The listing builds one solid part. Answer for the finished solid, in the listing's coordinates (mm). A direction names the side the tool comes from. Give positions to 0.01 mm unless a question says otherwise; leave off trailing zeros. Loops run counter-clockwise (first coordinate to the right, second up) from the corner with the lowest first, then second, coordinate; pieces in that order, holes last. Notation, with made-up numbers: (15, -13) - (49, -13) arc R19 ccw to (49, -2) - close; hole circle Ø7 at (-6, -32). An arc over 180 degrees is marked (long way). Write each question's results on one line, items separated by ' | '.
from build123d import *

# Parameters (mm, degrees)
SKETCH3_W           = 60
SKETCH3_H           = 80
SKETCH3_R           = 1
SKETCH3_R_2         = 1.5
SKETCH3_W_2         = 22
SKETCH3_H_2         = 45
BOSS_EXTRUDE1_DEPTH = 5
SKETCH4_W           = 32
SKETCH4_H           = 50
CUT_EXTRUDE1_DEPTH  = 2


with BuildPart() as part:
    # Sketch3 → Boss-Extrude1 (new body)
    with BuildSketch(Plane(origin=(0, 0, 0), x_dir=(1, 0, 0), z_dir=(0, 1, 0))):
        Rectangle(SKETCH3_W, SKETCH3_H)
        with Locations(Location((-13.5, 22.8, 0), (0, 0, 270))):
            Circle(SKETCH3_R, mode=Mode.SUBTRACT)
        with Locations(Location((13.5, 22.8, 0), (0, 0, 270))):
            Circle(SKETCH3_R, mode=Mode.SUBTRACT)
        with Locations(Location((-13.5, 14.8, 0), (0, 0, 270))):
            Circle(SKETCH3_R, mode=Mode.SUBTRACT)
        with Locations(Location((-13.5, 6.8, 0), (0, 0, 270))):
            Circle(SKETCH3_R, mode=Mode.SUBTRACT)
        with Locations(Location((13.5, 14.8, 0), (0, 0, 270))):
            Circle(SKETCH3_R, mode=Mode.SUBTRACT)
        with Locations(Location((13.5, 6.8, 0), (0, 0, 270))):
            Circle(SKETCH3_R, mode=Mode.SUBTRACT)
        with Locations(Location((-13.5, 30.8, 0), (0, 0, 270))):
            Circle(SKETCH3_R, mode=Mode.SUBTRACT)
        with Locations(Location((13.5, 30.8, 0), (0, 0, 270))):
            Circle(SKETCH3_R, mode=Mode.SUBTRACT)
        with Locations(Location((-25, 30, 0), (0, 0, 270))):
            Circle(SKETCH3_R_2, mode=Mode.SUBTRACT)
        with Locations(Location((25, 30, 0), (0, 0, 270))):
            Circle(SKETCH3_R_2, mode=Mode.SUBTRACT)
        with Locations(Location((-25, 10, 0), (0, 0, 270))):
            Circle(SKETCH3_R_2, mode=Mode.SUBTRACT)
        with Locations(Location((-25, -10, 0), (0, 0, 270))):
            Circle(SKETCH3_R_2, mode=Mode.SUBTRACT)
        with Locations(Location((-25, -30, 0), (0, 0, 270))):
            Circle(SKETCH3_R_2, mode=Mode.SUBTRACT)
        with Locations(Location((25, 10, 0), (0, 0, 270))):
            Circle(SKETCH3_R_2, mode=Mode.SUBTRACT)
        with Locations(Location((25, -10, 0), (0, 0, 270))):
            Circle(SKETCH3_R_2, mode=Mode.SUBTRACT)
        with Locations(Location((25, -30, 0), (0, 0, 270))):
            Circle(SKETCH3_R_2, mode=Mode.SUBTRACT)
        with Locations((0, 13)):
            Rectangle(SKETCH3_W_2, SKETCH3_H_2, mode=Mode.SUBTRACT)
    extrude(amount=BOSS_EXTRUDE1_DEPTH)

    # Sketch4 → Cut-Extrude1 (cut)
    with BuildSketch(Plane(origin=(0, 5, 0), x_dir=(1, 0, 0), z_dir=(0, 1, 0))):
        with Locations((0, 13.55)):
            Rectangle(SKETCH4_W, SKETCH4_H)
    extrude(amount=-CUT_EXTRUDE1_DEPTH, mode=Mode.SUBTRACT)


solid = part.part
Item 1: For a pull along X with two mould halves and no side action, classify faces 4 (the face through (0, 5, 17)), 5 (the face through (12.61, 1.48, -6.34)), 6 (the face through (30, 2, 1)), 7 (the face through (26.01, 2.46, 28.89)) as released by +X, released by -X, zero draft, split by the parting line, or undercut.
Values found:
face 4: zero draft | face 5: undercut | face 6: released by +X | face 7: undercut
Item 2: A cutting plane is placed at C-C, the plane z = 30. Determine the outline of the cut face in (x, y), plus the area to 3 significant figures.
Values found:
outline: (-30, 0) - (-26.5, 0) - (-26.5, 5) - (-30, 5) - close; (-23.5, 0) - (23.5, 0) - (23.5, 5) - (-23.5, 5) - close; (26.5, 0) - (30, 0) - (30, 5) - (26.5, 5) - close | area: 270 mm²
Item 3: A cutting plane is placed at A-A, the plane y = 1.15. Count the separate pieces of the cut face and the enclosed holes in it, plus the area to 3 significant figures.
Values found:
separate pieces: 1 | enclosed holes: 17 | area: 3,730 mm²
Item 4: A cutting plane is placed at D-D, the plane x = -13.5. Determine the outline of the cut face in (y, z), plus the area to 3 significant figures.
Values found:
outline: (0, -40) - (5, -40) - (5, -38.55) - (3, -38.55) - (3, -31.8) - (0, -31.8) - close; (0, -29.8) - (3, -29.8) - (3, -23.8) - (0, -23.8) - close; (0, -21.8) - (3, -21.8) - (3, -15.8) - (0, -15.8) - close; (0, -13.8) - (3, -13.8) - (3, -7.8) - (0, -7.8) - close; (0, -5.8) - (3, -5.8) - (3, 11.45) - (5, 11.45) - (5, 40) - (0, 40) - close | area: 276 mm²
Item 5: A cutting plane is placed at B-B, the plane x = -3. Determine the outline of the cut face in (y, z).
Values found:
outline: (0, -40) - (5, -40) - (5, -38.55) - (3, -38.55) - (3, -35.5) - (0, -35.5) - close; (0, 9.5) - (3, 9.5) - (3, 11.45) - (5, 11.45) - (5, 40) - (0, 40) - close
Item 6: Flat-ended cylindrical pins translate along their axes: P1, Ø2.5, axis at x = -13.5, z = -30.8, coming from the +Y side; P2, Ø4, axis at x = -19, z = 14.5, coming from the -Y side. Find the tip coordinate at first contact, or state that the pin passes through.
Values found:
P1: stops at y = 3 | P2: stops at y = 0
Item 7: Find the intervals of material crossed by line 1 along Z through (x, y) = (-13.5, 1.7); line 2 along X through (y, z) = (3.65, 0); line 3 along Z through (x, y) = (8.5, 3.05), in increasing order. Write a range as [from, to].
Values found:
line 1: z = [-40, -31.8], [-29.8, -23.8], [-21.8, -15.8], [-13.8, -7.8], [-5.8, 40] | line 2: x = [-30, -16], [16, 30] | line 3: z = [-40, -38.55], [11.45, 40]
Item 8: For faces 1 (the face through (0, 2, 40)), 2 (the face through (11, 1, -13)), 3 (the face through (0, 4, -38.55)), determine the directions among +Z, -Z, +X, -X, +Y, -Y from which every point of the face is accessible in a straight line to the end or side of a thin tool.
Values found:
face 1: +Z, +X, -X, +Y, -Y | face 2: +Y, -Y | face 3: +Y
